from build123d import *

# Parameters (mm, degrees)
SKETCH_1_W          = 95
SKETCH_1_H          = 178
EXTRUDE_1_DEPTH     = 160
SKETCH_2_W          = 145
SKETCH_2_H          = 26.5
SKETCH_2_W_2        = 185
CUT_EXTRUDE_1_DEPTH = 258.50533975
FILLET_1_R          = 62.5
SKETCH_3_R          = 50
CUT_EXTRUDE_2_DEPTH = 230
SKETCH_5_R          = 50
SKETCH_5_R_2        = 15
EXTRUDE_3_DEPTH     = 7
SKETCH_6_R          = 25
CUT_EXTRUDE_3_DEPTH = 40
SKETCH_11_R         = 2.5
CUT_EXTRUDE_4_DEPTH = 15
CUT_EXTRUDE_5_DEPTH = 40
SKETCH_13_R         = 3
CUT_EXTRUDE_6_DEPTH = 20
SKETCH_14_R         = 5
CUT_EXTRUDE_7_DEPTH = 40
FILLET_2_R          = 5


with BuildPart() as part:
    # 草图1 → 拉伸1 (new body)
    with BuildSketch(Plane.XY):
        with Locations((47.5, -89)):
            Rectangle(SKETCH_1_W, SKETCH_1_H)
    extrude(amount=EXTRUDE_1_DEPTH)

    # 草图2 → 切除-拉伸1 (cut, through all)
    with BuildSketch(Plane(origin=(95, 0, 0), x_dir=(0, 0, -1), z_dir=(1, 0, 0))):
        with Locations((-87.5, -164.75)):
            Rectangle(SKETCH_2_W, SKETCH_2_H)
        with Locations((-107.5, -13.25)):
            Rectangle(SKETCH_2_W_2, SKETCH_2_H)
    extrude(amount=-CUT_EXTRUDE_1_DEPTH, mode=Mode.SUBTRACT)

    # 圆角1
    fillet_1_edges = [part.edges().sort_by_distance(p)[0] for p in [
        (47.5, -26.5, 160),
        (47.5, -151.5, 160),
    ]]
    fillet(fillet_1_edges, radius=FILLET_1_R - 0.0001)  # a hair under: the kernel refuses the full size

    # 草图3 → 切除-拉伸2 (cut)
    with BuildSketch(Plane(origin=(95, 0, 0), x_dir=(0, 0, -1), z_dir=(1, 0, 0))):
        with Locations(Location((-97.5, -89, 0), (0, 0, 90))):
            Circle(SKETCH_3_R)
    extrude(amount=-CUT_EXTRUDE_2_DEPTH, mode=Mode.SUBTRACT)

    # 草图5 → 拉伸3 (add)
    with BuildSketch(Plane(origin=(95, 0, 0), x_dir=(0, 0, -1), z_dir=(1, 0, 0))):
        with Locations(Location((-97.5, -89, 0), (0, 0, 90))):
            Circle(SKETCH_5_R)
        with Locations(Location((-97.5, -89, 0), (0, 0, 90))):
            Circle(SKETCH_5_R_2, mode=Mode.SUBTRACT)
    extrude(amount=-EXTRUDE_3_DEPTH)

    # 草图6 → 切除-拉伸3 (cut)
    with BuildSketch(Plane(origin=(95, 0, 0), x_dir=(0, 0, -1), z_dir=(1, 0, 0))):
        with Locations(Location((-40.084300927, -58, 0), (0, 0, 165.276076349))):
            Circle(SKETCH_6_R)
    extrude(amount=-CUT_EXTRUDE_3_DEPTH, mode=Mode.SUBTRACT)

    # 草图11 → 切除-拉伸4 (cut)
    with BuildSketch(Plane(origin=(95, 0, 0), x_dir=(0, 0, -1), z_dir=(1, 0, 0))):
        with Locations(Location((-64.833038269, -82.748737342, 0), (0, 0, 90))):
            Circle(SKETCH_11_R)
        with Locations(Location((-64.833038269, -33.251262658, 0), (0, 0, 270))):
            Circle(SKETCH_11_R)
        with Locations(Location((-15.335563586, -33.251262658, 0), (0, 0, 270))):
            Circle(SKETCH_11_R)
        with Locations(Location((-15.335563586, -82.748737342, 0), (0, 0, 270))):
            Circle(SKETCH_11_R)
    extrude(amount=-CUT_EXTRUDE_4_DEPTH, mode=Mode.SUBTRACT)

    # 草图12 → 切除-拉伸5 (cut)
    with BuildSketch(Plane(origin=(0, 0, 0), x_dir=(-1, 0, 0), z_dir=(0, 0, -1))):
        Polygon((-45, -39), (-20, -39), (-20, -139), (-45, -139), (-75, -139), (-75, -89), (-45, -89), align=None)
    extrude(amount=-CUT_EXTRUDE_5_DEPTH, mode=Mode.SUBTRACT)

    # 草图13 → 切除-拉伸6 (cut)
    with BuildSketch(Plane.ZY):
        with Locations(Location((153.5, -89, 0), (0, 0, 270))):
            Circle(SKETCH_13_R)
        with Locations(Location((142.804951685, -121.915974128, 0), (0, 0, 270))):
            Circle(SKETCH_13_R)
        with Locations(Location((114.804951685, -142.259164913, 0), (0, 0, 270))):
            Circle(SKETCH_13_R)
        with Locations(Location((80.195048315, -142.259164913, 0), (0, 0, 270))):
            Circle(SKETCH_13_R)
        with Locations(Location((52.195048315, -121.915974128, 0), (0, 0, 270))):
            Circle(SKETCH_13_R)
        with Locations(Location((41.5, -89, 0), (0, 0, 270))):
            Circle(SKETCH_13_R)
        with Locations(Location((52.195048315, -56.084025872, 0), (0, 0, 270))):
            Circle(SKETCH_13_R)
        with Locations(Location((80.195048315, -35.740835087, 0), (0, 0, 270))):
            Circle(SKETCH_13_R)
        with Locations(Location((114.804951685, -35.740835087, 0), (0, 0, 270))):
            Circle(SKETCH_13_R)
        with Locations(Location((142.804951685, -56.084025872, 0), (0, 0, 270))):
            Circle(SKETCH_13_R)
    extrude(amount=-CUT_EXTRUDE_6_DEPTH, mode=Mode.SUBTRACT)

    # 草图14 → 切除-拉伸7 (cut)
    with BuildSketch(Plane.XY.offset(15)):
        with Locations((12.5, -164)):
            Circle(SKETCH_14_R)
        with Locations((47.5, -164)):
            Circle(SKETCH_14_R)
        with Locations((82.5, -164)):
            Circle(SKETCH_14_R)
        with Locations((12.5, -14)):
            Circle(SKETCH_14_R)
        with Locations((47.5, -14)):
            Circle(SKETCH_14_R)
        with Locations((82.5, -14)):
            Circle(SKETCH_14_R)
    extrude(amount=-CUT_EXTRUDE_7_DEPTH, mode=Mode.SUBTRACT)

    # 圆角2
    fillet_2_edges = [part.edges().sort_by_distance(p)[0] for p in [
        (47.5, -151.5, 15),
        (47.5, -26.5, 15),
    ]]
    fillet(fillet_2_edges, radius=FILLET_2_R)


solid = part.part
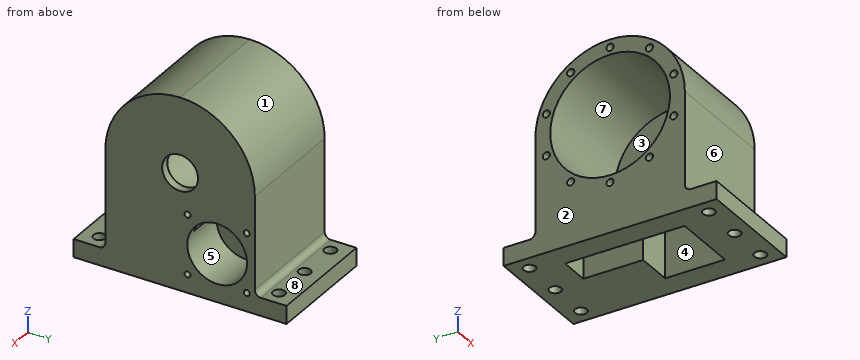
Source: CAD feature listing. Evaluate the final solid. Frame: model axes, mm. Face numbers are marked on the shaded views. A direction names the side the tool comes from. Give positions to 0.01 mm unless a question says otherwise; leave off trailing zeros. Write each loop counter-clockwise with the first axis right and the second up, starting at its lowest first coordinate (ties: lowest second). Pieces come first, ordered by that corner, then holes. Notation, with made-up numbers: (76.5, -37.5) -> (113.5, -37.5) arc R13 cw to (113.5, -13.5) -> close; hole circle Ø3 at (-32, -38). An arc over 180 degrees is marked (long way). Write item = value, one per line.
Q1. Cut plane A-A on x = 47.5. State how many separate pieces and enclosed holes the cut face has, then the cut area to 3 significant figures.
Here are the results:
separate_pieces = 3
enclosed_holes = 1
area = 8,980 mm²
Q2. Line query: line 1 (Y direction, x = 82.5, z = 12); line 2 (Y direction, x = 63.5, z = 21); line 3 (Z direction, x = 91, y = -89). Output: solid intervals per line, ascending. Write a range as from..to.
Here are the results:
line_1 = -178..-169, -159..-19, -9..0
line_2 = -151.5..-139, -89..-74.15, -41.85..-26.5
line_3 = 0..82.5, 112.5..160
Q3. First-contact query: pin 1 (10 mm diameter, centred on x = 52.5, z = 113, fed in from -Y); pin 2 (2 mm diameter, centred on x = 77.5, z = 103, fed in from +Y); pin 3 (3 mm diameter, centred on x = 25.5, y = -76.5, fed in from -Z). Flat tips, straight axial feed; report the tip coordinate or a pass-through.
Here are the results:
pin_1 = -150.61
pin_2 = -26.66
pin_3 = 40
Q4. Mould query, pull axis Y, two halves, no side actions, for the marked faces 1, 2 and 3. Classes: +Y half, -Y half, draft (parallel to the pull), parting line (faces both ways), or undercut.
Here are the results:
face_1 = +Y half
face_2 = draft
face_3 = undercut
Q5. Reachability of the marked faces 4, 5, 6, 7 and 8 from +Z, -Z, +X, -X, +Y, -Y: full face, straight path, thin tool, end or side. Return the list, or none.
Here are the results:
face_4 = -Z
face_5 = +X
face_6 = +Z, +X, -X, -Y
face_7 = -X
face_8 = +Z, +X, -X, +Y
Q6. Cut plane B-B on y = -164. Return loops of the section in (x, z).
Here are the results:
outline = (0, 0) -> (7.5, 0) -> (7.5, 15) -> (0, 15) -> close; (17.5, 0) -> (42.5, 0) -> (42.5, 15) -> (17.5, 15) -> close; (52.5, 0) -> (77.5, 0) -> (77.5, 15) -> (52.5, 15) -> close; (87.5, 0) -> (95, 0) -> (95, 15) -> (87.5, 15) -> close
